The listing builds one solid part. Answer for the finished solid, in the listing's coordinates (mm). Face numbers are marked on the shaded views. A direction names the side the tool comes from. Round coordinates to 2 decimals unless told otherwise and drop trailing zeros. Order: outer loops, then holes, each group sorted by start corner. A loop starts at its lowest first (then second) coordinate and runs counter-clockwise, first axis right, second up. Notation, with made-up numbers: (55, -31.75) - (96, -31.75) arc R23 cw to (96, -7.75) - close; hole circle Ø6 at (10, 56). An arc over 180 degrees is marked (long way). One line per item, written item: value. Start each with the question number.
1. Straight lines are drawn through the part: line 1 (X direction, y = -87, z = -85.5); line 2 (Z direction, x = -273.5, y = 631); line 3 (X direction, y = 571.5, z = -5.5). For each, find the intervals that lie inside material, in ascending order.
2. Section C-C, the plane y = 1121.5 is taken. Give the vertices of the cut face in (x, z), then the cut area to 3 significant figures.
3. Section A-A, the plane x = -287 is taken. Give the vertices of the cut face in (y, z).
4. Section B-B, the plane x = 154.5 is taken. Give the vertices of the cut face in (y, z), then the cut area to 3 significant figures.
5. A tool of negligible diameter and unlimited length cuts with its end or side. For the marked faces 1, 2 and 3, from which of +Z, -Z, +X, -X, +Y, -Y can it reach the whole face along a straight path? Write none if from no direction.
6. Section D-D, the plane z = -336.5 is taken. Give the vertices of the cut face in (x, y), then the cut area to 3 significant figures.
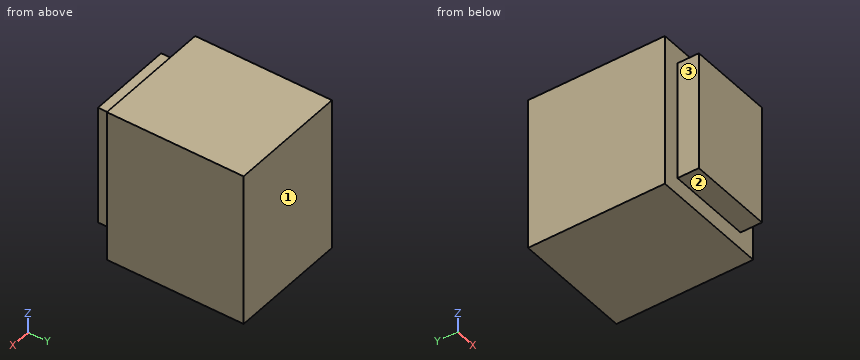
from build123d import *

# Parameters (mm, degrees)
SKETCH1_W           = 1400
SKETCH1_H           = 1800
BOSS_EXTRUDE1_DEPTH = 1600
SKETCH2_W           = 1000
SKETCH2_H           = 1400
BOSS_EXTRUDE2_DEPTH = 250
SKETCH3_W           = 800
SKETCH3_H           = 1000
CUT_EXTRUDE1_DEPTH  = 50
SKETCH4_W           = 500
SKETCH4_H           = 350
BOSS_EXTRUDE3_DEPTH = 50


with BuildPart() as part:
    # Sketch1 → Boss-Extrude1 (new body)
    with BuildSketch(Plane(origin=(0, 0, 0), x_dir=(1, 0, 0), z_dir=(0, 1, 0))):
        Rectangle(SKETCH1_W, SKETCH1_H)
    extrude(amount=BOSS_EXTRUDE1_DEPTH)

    # Sketch2 → Boss-Extrude2 (add)
    with BuildSketch(Plane(origin=(0, 0, 0), x_dir=(1, 0, 0), z_dir=(0, 1, 0))):
        Rectangle(SKETCH2_W, SKETCH2_H)
    extrude(amount=-BOSS_EXTRUDE2_DEPTH)

    # Sketch3 → Cut-Extrude1 (cut)
    with BuildSketch(Plane.XY):
        with Locations((7.862922359, 800.806757739)):
            Rectangle(SKETCH3_W, SKETCH3_H)
    extrude(amount=-CUT_EXTRUDE1_DEPTH, mode=Mode.SUBTRACT)

    # Sketch4 → Boss-Extrude3 (add)
    with BuildSketch(Plane.XY):
        with Locations((23.588767076, 824.395524815)):
            Rectangle(SKETCH4_W, SKETCH4_H)
    extrude(amount=-BOSS_EXTRUDE3_DEPTH)


solid = part.part
Answer list:
1. line 1: x = -500 to 500
1. line 2: z = -900 to -50, 0 to 900
1. line 3: x = -700 to -392.14, 407.86 to 700
2. outline: (-700, -900) - (700, -900) - (700, 900) - (-700, 900) - close; hole (-392.14, -50) - (407.86, -50) - (407.86, 0) - (-392.14, 0) - close
2. area: 2,480,000 mm²
3. outline: (-250, -700) - (0, -700) - (0, -900) - (1600, -900) - (1600, 900) - (0, 900) - (0, 700) - (-250, 700) - close; hole (300.81, -50) - (1300.81, -50) - (1300.81, 0) - (300.81, 0) - close
4. outline: (-250, -700) - (0, -700) - (0, -900) - (1600, -900) - (1600, 900) - (0, 900) - (0, 700) - (-250, 700) - close; hole (300.81, -50) - (649.4, -50) - (649.4, 0) - (300.81, 0) - close; hole (999.4, -50) - (1300.81, -50) - (1300.81, 0) - (999.4, 0) - close
4. area: 3,200,000 mm²
5. face 1: +Z, -Z, +X, -X, +Y
5. face 2: -Z, +X, -X, -Y
5. face 3: +Z, -Z, -X, -Y
6. outline: (-700, 0) - (-500, 0) - (-500, -250) - (500, -250) - (500, 0) - (700, 0) - (700, 1600) - (-700, 1600) - close
6. area: 2,490,000 mm²
